```python
from build123d import *

# Parameters (mm, degrees)
F2_START = 1.6
F2_DEPTH = 4.9
F3_W     = 2
F3_H     = 5.2
F4_DEPTH = 5.95
F5_W     = 13
F5_H     = 3
F6_DEPTH = 12.5
F7_R     = 1.85
F8_DEPTH = 6


with BuildPart() as f2:
    # F1 (on Top) → F2 (new body)
    with BuildSketch(Plane.XY.offset(F2_START)):
        with BuildLine():
            ThreePointArc((20.5, 5.5), (19.0355339059, 9.0355339059), (15.5, 10.5))
            Line((15.5, 10.5), (-15.5, 10.5))
            ThreePointArc((-15.5, 10.5), (-19.0355339059, 9.0355339059), (-20.5, 5.5))
            Line((-20.5, 5.5), (-20.5, -5.5))
            ThreePointArc((-20.5, -5.5), (-19.0355339059, -9.0355339059), (-15.5, -10.5))
            Line((-15.5, -10.5), (15.5, -10.5))
            ThreePointArc((15.5, -10.5), (19.0355339059, -9.0355339059), (20.5, -5.5))
            Line((20.5, -5.5), (20.5, 5.5))
        make_face()
    extrude(amount=F2_DEPTH)

    # F3 (on Front) → F4 (cut, symmetric)
    with BuildSketch(Plane.XZ):
        with BuildLine():
            ThreePointArc((3.6728735344, -2.6), (4.2882357039, -1.3641974005), (4.5, 0))
            ThreePointArc((4.5, 0), (4.2882357039, 1.3641974005), (3.6728735344, 2.6))
            Line((3.6728735344, 2.6), (-3.6728735344, 2.6))
            ThreePointArc((-3.6728735344, 2.6), (-4.5, 0), (-3.6728735344, -2.6))
            Line((-3.6728735344, -2.6), (3.6728735344, -2.6))
        make_face()
        with BuildLine():
            ThreePointArc((3.6728735344, 2.6), (4.2882357039, 1.3641974005), (4.5, 0))
            ThreePointArc((4.5, 0), (4.2882357039, -1.3641974005), (3.6728735344, -2.6))
            Line((3.6728735344, -2.6), (8, -2.6))
            Line((8, -2.6), (8, 2.6))
            Line((8, 2.6), (3.6728735344, 2.6))
        make_face()
        with BuildLine():
            Line((-3.6728735344, 2.6), (3.6728735344, 2.6))
            ThreePointArc((3.6728735344, 2.6), (0, 4.5), (-3.6728735344, 2.6))
        make_face()
        with BuildLine():
            ThreePointArc((-3.6728735344, -2.6), (0, -4.5), (3.6728735344, -2.6))
            Line((3.6728735344, -2.6), (-3.6728735344, -2.6))
        make_face()
        with BuildLine():
            ThreePointArc((-3.6728735344, -2.6), (-4.5, 0), (-3.6728735344, 2.6))
            Line((-3.6728735344, 2.6), (-8, 2.6))
            Line((-8, 2.6), (-8, -2.6))
            Line((-8, -2.6), (-3.6728735344, -2.6))
        make_face()
        with Locations((-9, 0)):
            Rectangle(F3_W, F3_H)
    extrude(amount=F4_DEPTH, both=True, mode=Mode.SUBTRACT)

    # F5 (on Front) → F6 (cut, symmetric)
    with BuildSketch(Plane.XZ):
        Rectangle(F5_W, F5_H)
    extrude(amount=F6_DEPTH, both=True, mode=Mode.SUBTRACT)

    # F7 (on face) → F8 (cut)
    with BuildSketch(Plane(origin=(0, 0, 1.6), x_dir=(1, 0, 0), z_dir=(0, 0, -1))):
        with Locations((-12.5, 0)):
            Circle(F7_R)
        with Locations((12.5, 0)):
            Circle(F7_R)
    extrude(amount=-F8_DEPTH, mode=Mode.SUBTRACT)


solid = f2.part
```
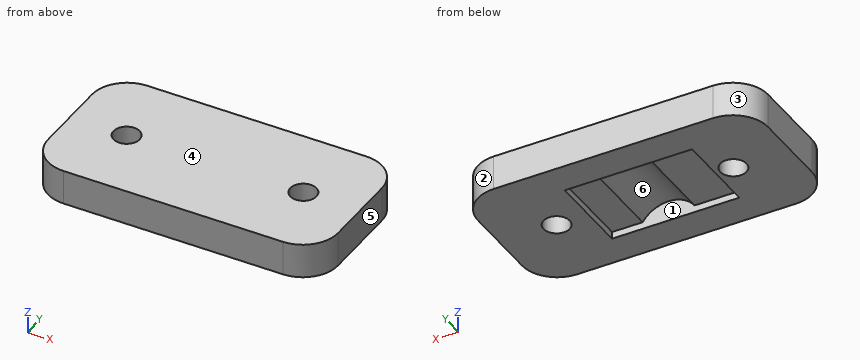
Here's how the part is built. I have some questions about the finished solid (model axes, mm). Face numbers are marked on the shaded views. A direction names the side the tool comes from. Give positions to 0.01 mm unless a question says otherwise; leave off trailing zeros. Write each loop counter-clockwise with the first axis right and the second up, starting at its lowest first coordinate (ties: lowest second). Pieces come first, ordered by that corner, then holes.
(1) If I drill on L1, parallel to X at y = 0, z = 4.1; L2, parallel to Y at x = 12.5, z = 3.3; L3, parallel to X at y = 0, z = 2.8, over which ranges is the centre line in solid material (lowest first)?
Output values:
L1: x = -20.5 to -14.35, -10.65 to -1.85, 1.85 to 10.65, 14.35 to 20.5
L2: y = -10.5 to -1.85, 1.85 to 10.5
L3: x = -20.5 to -14.35, -10.65 to -3.52, 3.52 to 10.65, 14.35 to 20.5
(2) Imagine slicing it at D-D, the plane z = 3.45. Write out the boundary of the cut face in (x, y), and give its area (3 significant figures).
Output values:
outline: (-20.5, -5.5) arc R5 ccw to (-15.5, -10.5) - (15.5, -10.5) arc R5 ccw to (20.5, -5.5) - (20.5, 5.5) arc R5 ccw to (15.5, 10.5) - (-15.5, 10.5) arc R5 ccw to (-20.5, 5.5) - close; hole circle Ø3.7 at (-12.5, 0); hole (-2.89, -5.95) - (2.89, -5.95) - (2.89, 5.95) - (-2.89, 5.95) - close; hole circle Ø3.7 at (12.5, 0)
area: 749 mm2
(3) Thinking about a two-plate mould opening in X: for the marked faces 1, 2, 3 and 4, which applies, pulls with the +X half, pulls with the -X half, needs draft (parallel to the pull), parting line crosses it, or undercut?
Output values:
face 1: undercut
face 2: pulls with the +X half
face 3: pulls with the -X half
face 4: needs draft
(4) Imagine slicing it at B-B, the plane x = -12.5. Write out the boundary of the cut face in (y, z).
Output values:
outline: (-10.5, 1.6) - (-1.85, 1.6) - (-1.85, 6.5) - (-10.5, 6.5) - close; (1.85, 1.6) - (10.5, 1.6) - (10.5, 6.5) - (1.85, 6.5) - close
(5) On a 3-axis mill with a long thin cutter (end or side, diameter ignored), from which of +Z, -Z, +X, -X, +Y, -Y can I reach the whole of each face in a straight line? I mean the marked faces 5 and 6. Say none if no direction works.
Output values:
face 5: +Z, -Z, +X, +Y, -Y
face 6: -Z
(6) Imagine slicing it at C-C, the plane z = 5.1. Write out the boundary of the cut face in (x, y), and give its area (3 significant figures).
Output values:
outline: (-20.5, -5.5) arc R5 ccw to (-15.5, -10.5) - (15.5, -10.5) arc R5 ccw to (20.5, -5.5) - (20.5, 5.5) arc R5 ccw to (15.5, 10.5) - (-15.5, 10.5) arc R5 ccw to (-20.5, 5.5) - close; hole circle Ø3.7 at (-12.5, 0); hole circle Ø3.7 at (12.5, 0)
area: 818 mm2
(7) Will these pins go through, and if not, where does the flat tip stop? pin 1 (3 mm diameter, centred on x = -7.5, y = 0, fed in from -Z); pin 2 (2 mm diameter, centred on x = -12.5, y = 0, fed in from +Z).
Output values:
pin 1: stops at z = 2.6
pin 2: passes through
(8) Imagine slicing it at A-A, the plane y = 0. Write out the boundary of the cut face in (x, z).
Output values:
outline: (-20.5, 1.6) - (-14.35, 1.6) - (-14.35, 6.5) - (-20.5, 6.5) - close; (-10.65, 1.6) - (-10, 1.6) - (-10, 2.6) - (-3.67, 2.6) arc R4.5 cw to (3.67, 2.6) - (8, 2.6) - (8, 1.6) - (10.65, 1.6) - (10.65, 6.5) - (-10.65, 6.5) - close; (14.35, 1.6) - (20.5, 1.6) - (20.5, 6.5) - (14.35, 6.5) - close
